Build history of the part. All positions in model axes, mm. Round coordinates to 2 decimals unless told otherwise and drop trailing zeros. Order: outer loops, then holes, each group sorted by start corner. A loop starts at its lowest first (then second) coordinate and runs counter-clockwise, first axis right, second up. Notation, with made-up numbers: (16, 78.5) - (71, 78.5) arc R28 cw to (71, 109.5) - close; hole circle Ø11 at (36, 87). An arc over 180 degrees is marked (long way). Write each question's results on one line, items separated by ' | '. Start each with the question number.
```python
from build123d import *

# Parameters (mm, degrees)
ESQUISSE1_R        = 1.6
BOSS_EXTRU_1_DEPTH = 1.55
CONG_1_R           = 0.7


with BuildPart() as part:
    # Esquisse1 → Boss.-Extru.1 (new body)
    with BuildSketch(Plane(origin=(0, 0, 0), x_dir=(1, 0, 0), z_dir=(0, 1, 0))):
        Polygon((65.7, 53.05), (65.7, 40.2), (68.2, 37.7), (68.2, 4.8), (65.7, 2.3), (65.7, 0), (0, 0), (0, 53.05), align=None)
        with Locations((15, 50.7)):
            Circle(ESQUISSE1_R, mode=Mode.SUBTRACT)
        with Locations((13.6, 2.4)):
            Circle(ESQUISSE1_R, mode=Mode.SUBTRACT)
        with Locations((65.8, 7.6)):
            Circle(ESQUISSE1_R, mode=Mode.SUBTRACT)
        with Locations((65.8, 35.55)):
            Circle(ESQUISSE1_R, mode=Mode.SUBTRACT)
    extrude(amount=BOSS_EXTRU_1_DEPTH)

    # Congé1
    cong_1_edges = [part.edges().sort_by_distance(p)[0] for p in [
        (0, 0.775, -53.05),
        (65.7, 0.775, -40.2),
        (65.7, 0.775, -2.3),
        (65.7, 0.775, 0),
        (0, 0.775, 0),
    ]]
    fillet(cong_1_edges, radius=CONG_1_R)


solid = part.part
```
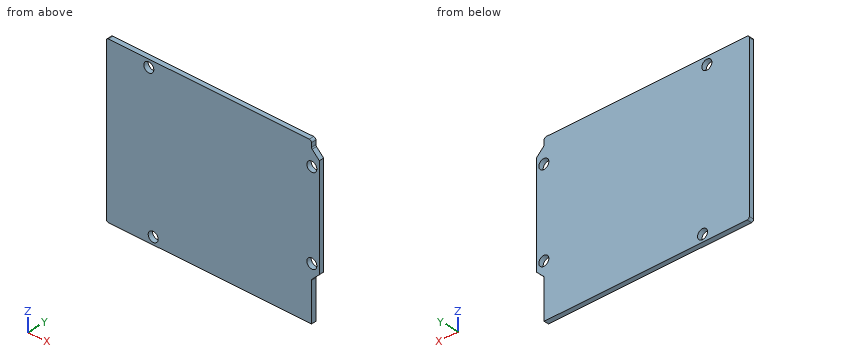
1. Cut at A-A (z = -50.7). List the corners of the cut face in (x, y).
2. Flat gauge pin, fed straight in: pin 1 Ø0.7 at (y, z) = (0.5, -1) entering from +X. Where does the tip first touch, or does it go through?
3. Cut at B-B (y = 1.15). List the corners of the cut face in (x, z).
4. Cut at C-C (z = -7.6). List the corners of the cut face in (x, y).
5. Wall check: line 1 (X direction, y = 1.2, z = -35.55); line 2 (Z direction, x = 13.6, y = 0.8); line 3 (X direction, y = 0.75, z = -50.7). Give the ranges that are in metal, low to high. Write a range as from..to.
A:
1) outline: (0, 0) - (13.4, 0) - (13.4, 1.55) - (0, 1.55) - close; (16.6, 0) - (65.7, 0) - (65.7, 1.55) - (16.6, 1.55) - close
2) pin 1: stops at x = 65.7
3) outline: (0, -52.35) arc R0.7 ccw to (0.7, -53.05) - (65.7, -53.05) - (65.7, -40.49) arc R0.7 cw to (65.91, -39.99) - (68.2, -37.7) - (68.2, -4.8) - (65.91, -2.51) arc R0.7 cw to (65.7, -2.01) - (65.7, -0.7) arc R0.7 ccw to (65, 0) - (0.7, 0) arc R0.7 ccw to (0, -0.7) - close; hole circle Ø3.2 at (13.6, -2.4); hole circle Ø3.2 at (15, -50.7); hole circle Ø3.2 at (65.8, -35.55); hole circle Ø3.2 at (65.8, -7.6)
4) outline: (0, 0) - (64.2, 0) - (64.2, 1.55) - (0, 1.55) - close; (67.4, 0) - (68.2, 0) - (68.2, 1.55) - (67.4, 1.55) - close
5) line 1: x = 0..64.2, 67.4..68.2 | line 2: z = -53.05..-51.47, -49.93..-4, -0.8..0 | line 3: x = 0..13.4, 16.6..65.7
